Input: part model. Units: mm. Frame: model coordinates. Face numbers are marked on the shaded views. A direction names the side the tool comes from. Round coordinates to 2 decimals unless told otherwise and drop trailing zeros. Loops run counter-clockwise (first coordinate to the right, second up) from the corner with the lowest first, then second, coordinate; pieces in that order, holes last. Notation, with made-up numbers: M -3.75,13.25 L 12.25,13.25 A21 ccw 12.25,30.25 Z; hole C 6.25,62 d3. An arc over 180 degrees is marked long. Return JSON: item names as keys, results as strings. Group by question number.
1) Section A-A (z = 0). Output: boundary loops of the cut face in (x, y), plus the area to 3 significant figures.
2) Section B-B (x = 0). Output: boundary loops of the cut face in (y, z).
3) Section D-D (y = -63). Output: boundary loops of the cut face in (x, z), plus the area to 3 significant figures.
4) Section C-C (y = -8.5). Output: boundary loops of the cut face in (x, z), plus the area to 3 significant figures.
5) Contact query for flat-ended pins moving along their axis: P1, Ø1, axis at y = -36.5, z = 7.5, coming from the +X side; P2, Ø9.5, axis at x = 0, z = 0, coming from the -Y side; P3, Ø8, axis at y = -44.5, z = -8, coming from the +X side; P4, Ø2, axis at y = -37.5, z = -2, coming from the -X side. Output: stop coordinate, or through.
6) Mould query, pull axis X, two halves, no side actions, for the marked faces 3 and 4. Classes: +X half, -X half, draft (parallel to the pull), parting line (faces both ways), or undercut.
7) Access query for the marked faces 1 and 2. Directions: +Z, -Z, +X, -X, +Y, -Y. A direction counts if a zero-diameter tool reaches every point of the face in a straight line with its end or side. Return the directions, or none.
8) Material intervals for line 1 (Z direction, x = 0, y = -46); line 2 (Z direction, x = 22, y = -5); line 3 (X direction, y = -14, z = 29.5), sorted ascending. Write a range as from..to.
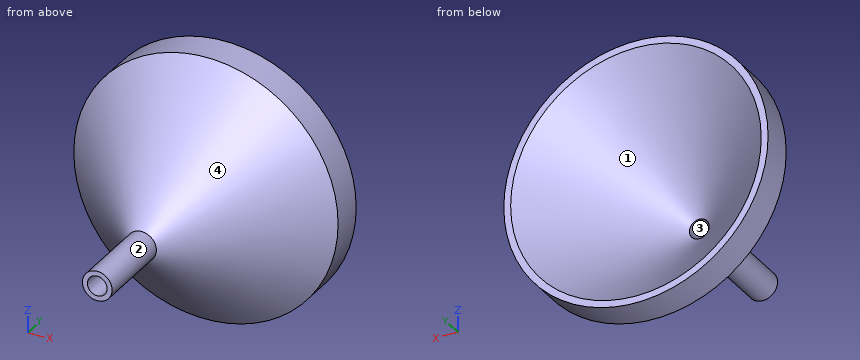
from build123d import *

# Parameters (mm, degrees)
F0_R     = 40.076976351
F0_R_2   = 4.5
F1_DEPTH = 50
F0_R_3   = 3
F3_DEPTH = 70
F4_SIZE  = 35


# Not quite as in the source:
# - a fillet or chamfer that OpenCascade refuses, or shapes differently, is made with other operations: its cross-section is extruded or revolved along the edge and cut away or added


with BuildPart() as f1:
    # F0 (on Front) → F1 (new body)
    with BuildSketch(Plane.XZ):
        Circle(F0_R)
        Circle(F0_R_2, mode=Mode.SUBTRACT)
    extrude(amount=F1_DEPTH)

    # F2: chamfer of 40 on 1 edges, made by hand

    # F2_s1 → F2_t2 (revolve, cut)
    with BuildSketch(Plane.XY):
        Polygon((40.076976351, -10), (0.076976351, -50), (40.076976351, -50), align=None)
    revolve(axis=Axis((0, -50, 0), (0, -1, 0)), mode=Mode.SUBTRACT)

    # F0 (on Front) → F3 (join)
    with BuildSketch(Plane.XZ):
        Circle(F0_R_2)
        Circle(F0_R_3, mode=Mode.SUBTRACT)
    extrude(amount=F3_DEPTH)

    # F4
    f4_edges = [f1.edges().sort_by_distance(p)[0] for p in [
        (-3, 0, 0),
    ]]
    chamfer(f4_edges, length=F4_SIZE)


solid = f1.part
Returned:
{
 "1": {"outline": "M -40.08,-10 L -4.5,-45.58 L -4.5,-70 L -3,-70 L -3,-35 L -38,0 L -40.08,0 Z; M 3,-70 L 4.5,-70 L 4.5,-45.58 L 40.08,-10 L 40.08,0 L 38,0 L 3,-35 Z", "area": "962 mm^2"},
 "2": {"outline": "M -70,-4.5 L -45.58,-4.5 L -10,-40.08 L 0,-40.08 L 0,-38 L -35,-3 L -70,-3 Z; M -70,3 L -35,3 L 0,38 L 0,40.08 L -10,40.08 L -45.58,4.5 L -70,4.5 Z"},
 "3": {"outline": "C 0,0 d9; hole C 0,0 d6", "area": "35.3 mm^2"},
 "4": {"outline": "C 0,0 d80.15; hole C 0,0 d59", "area": "2,310 mm^2"},
 "5": {"P1": "stops at x = 11.99", "P2": "stops at y = -70", "P3": "stops at x = 6.77", "P4": "stops at x = -13.44"},
 "6": {"face 3": "undercut", "face 4": "parting line"},
 "7": {"face 1": "+Y", "face 2": "-Y"},
 "8": {"line 1": "z = -4.5..-3, 3..4.5", "line 2": "z = -33.5..-24.6, 24.6..33.5", "line 3": "x = -20.77..20.77"}
}
